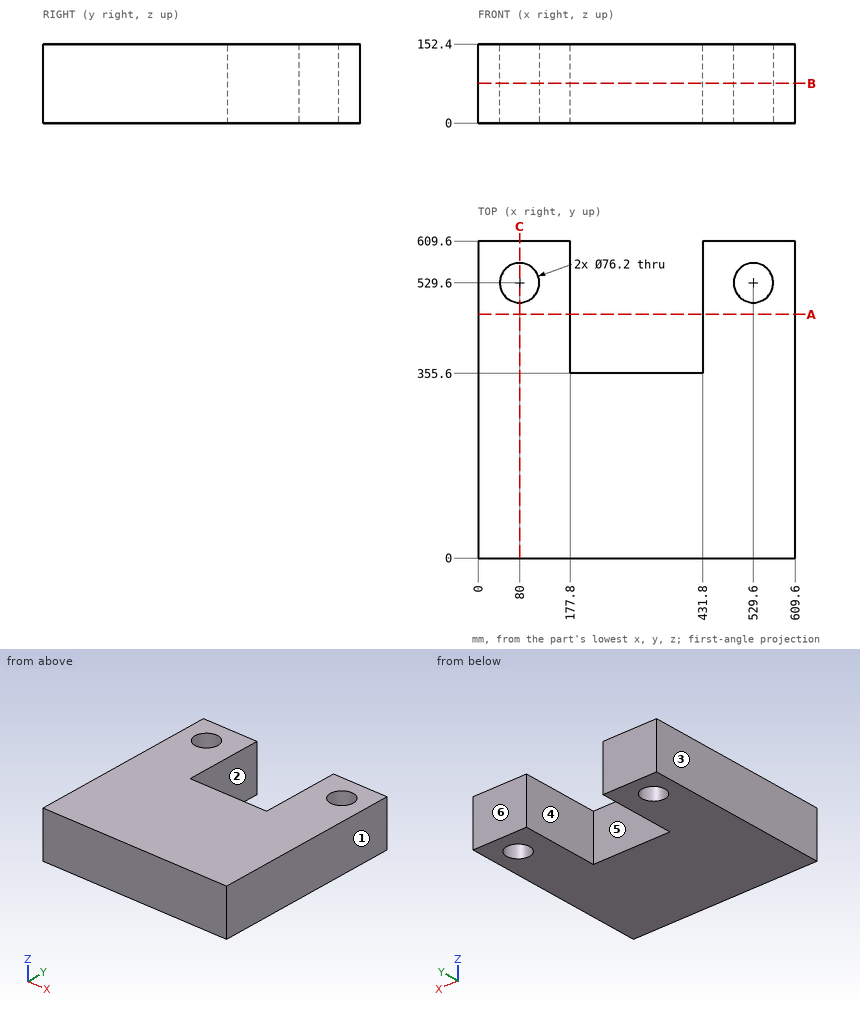
Source: three-view drawing plus pictorial views. Frame: mm from the lowest corner of the part. A direction names the side the tool comes from. Give positions to 0.01 mm unless a question says otherwise; leave off trailing zeros. Loops run counter-clockwise (first coordinate to the right, second up) from the corner with the lowest first, then second, coordinate; pieces in that order, holes last.
1) Line query: L1, parallel to X at y = 529.6, z = 59.5; L2, parallel to X at y = 407, z = 72; L3, parallel to Y at x = 80, z = 59. Output: solid intervals per line, ascending.
A:
L1: x = 0 to 41.9, 118.1 to 177.8, 431.8 to 491.5, 567.7 to 609.6
L2: x = 0 to 177.8, 431.8 to 609.6
L3: y = 0 to 491.5, 567.7 to 609.6
2) Section query B-B on z = 76.5. Return the cut outline in (x, y).
A:
outline: (0, 0) - (609.6, 0) - (609.6, 609.6) - (431.8, 609.6) - (431.8, 355.6) - (177.8, 355.6) - (177.8, 609.6) - (0, 609.6) - close; hole circle Ø76.2 at (80, 529.6); hole circle Ø76.2 at (529.6, 529.6)
3) Section query A-A on y = 469. Return the cut outline in (x, z).
A:
outline: (0, 0) - (177.8, 0) - (177.8, 152.4) - (0, 152.4) - close; (431.8, 0) - (609.6, 0) - (609.6, 152.4) - (431.8, 152.4) - close
4) Contact query for flat-ended pins moving along their axis: pin 1 (8 mm diameter, centred on x = 246, z = 117, fed in from +Y); pin 2 (8 mm diameter, centred on x = 491.5, y = 390, fed in from -Z). Output: stop coordinate, or through.
A:
pin 1: stops at y = 355.6
pin 2: stops at z = 0
5) Reachability of the marked faces 1 and 2 from +Z, -Z, +X, -X, +Y, -Y: full face, straight path, thin tool, end or side. Return the list, or none.
A:
face 1: +Z, -Z, +X, +Y, -Y
face 2: +Z, -Z, +Y
6) Section query C-C on x = 80. Return the cut outline in (y, z), and give its area (3 significant figures).
A:
outline: (0, 0) - (491.5, 0) - (491.5, 152.4) - (0, 152.4) - close; (567.7, 0) - (609.6, 0) - (609.6, 152.4) - (567.7, 152.4) - close
area: 81,300 mm2
7) Mould query, pull axis X, two halves, no side actions, for the marked faces 3, 4, 5 and 6. Classes: released by +X, released by -X, zero draft, split by the parting line, or undercut.
A:
face 3: released by -X
face 4: undercut
face 5: undercut
face 6: zero draft
